The model under review builds one solid part; all positions refer to its coordinate system, in mm. Face numbers are marked on the shaded views. A direction names the side the tool comes from. Coordinates: 2 decimals unless noted, no trailing zeros. Order: outer loops, then holes, each group sorted by start corner. A loop starts at its lowest first (then second) coordinate and runs counter-clockwise, first axis right, second up.
```python
from build123d import *

# Parameters (mm, degrees)
F0_W     = 15
F0_H     = 9.5
F1_DEPTH = 22
F0_W_2   = 8.7
F0_H_2   = 2.8
F2_DEPTH = 12
F3_R     = 1.5


with BuildPart() as f1:
    # F0 (on Top) → F1 (new body)
    with BuildSketch(Plane.XY):
        with Locations((0, 0.571325)):
            Rectangle(F0_W, F0_H)
        Polygon((5.5, 2.5), (5.5, -2.5), (-5.5, -2.5), (-5.5, 2.5), (-1.25, 2.5), (-1.25, 4.012365), (1.25, 4.012365), (1.25, 2.5), align=None, mode=Mode.SUBTRACT)
    extrude(amount=F1_DEPTH)

    # F0 (on Top) → F2 (join)
    with BuildSketch(Plane.XY):
        Polygon((-5.5, -2.5), (5.5, -2.5), (5.5, 2.5), (1.25, 2.5), (1.25, 4.012365), (-1.25, 4.012365), (-1.25, 2.5), (-5.5, 2.5), align=None)
        Rectangle(F0_W_2, F0_H_2, mode=Mode.SUBTRACT)
    extrude(amount=F2_DEPTH)

    # F3
    f3_edges = [f1.edges().sort_by_distance(p)[0] for p in [
        (-7.5, 5.321325, 11),
        (7.5, 5.321325, 11),
        (7.5, -4.178675, 11),
        (-7.5, -4.178675, 11),
    ]]
    fillet(f3_edges, radius=F3_R)


solid = f1.part
```
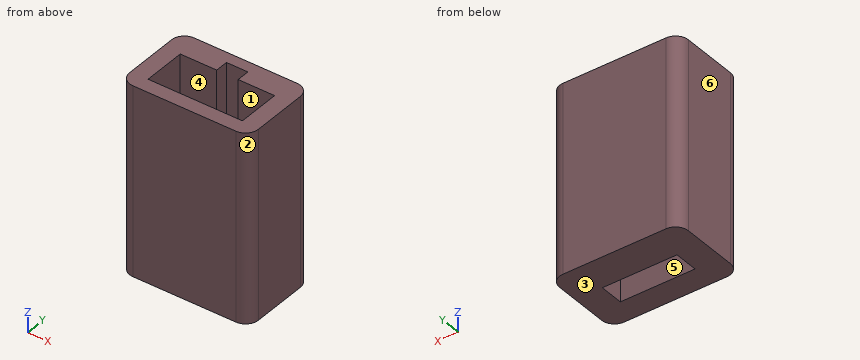
(1) We need section D-D, the plane y = 3. Write out the cut boundary in (x, z).
A:
outline: (-7.5, 0) - (7.5, 0) - (7.5, 22) - (1.25, 22) - (1.25, 12) - (-1.25, 12) - (-1.25, 22) - (-7.5, 22) - close
(2) Wall thickness on probe 1 along X at (y, z) = (-1.25, 14); probe 2 along Y at (x, z) = (-3.25, 11.5); probe 3 along Y at (x, z) = (-1.75, 20.75): over which ranges is each line inside the solid? List them lowest first.
A:
probe 1: x = -7.5 to -5.5, 5.5 to 7.5
probe 2: y = -4.18 to -1.4, 1.4 to 5.32
probe 3: y = -4.18 to -2.5, 2.5 to 5.32
(3) For pin 1 Ø3.5 at (x, y) = (1, 0) entering from +Z, flat-tipped, find the tip position at first contact; note if it passes through.
A:
pin 1: stops at z = 12
(4) Draft analysis for pull direction X (two halves, no side actions). For the marked faces 1, 2 and 3, state which applies: released by +X, released by -X, zero draft, split by the parting line, or undercut.
A:
face 1: undercut
face 2: released by +X
face 3: zero draft
(5) We need section A-A, the plane x = 1.5. Write out the cut boundary in (y, z), and give its area (3 significant figures).
A:
outline: (-4.18, 0) - (-1.4, 0) - (-1.4, 12) - (-2.5, 12) - (-2.5, 22) - (-4.18, 22) - close; (1.4, 0) - (5.32, 0) - (5.32, 22) - (2.5, 22) - (2.5, 12) - (1.4, 12) - close
area: 125 mm2
(6) Machinability: for the marked faces 4, 5 and 6, which of the approach directions +Z, -Z, +X, -X, +Y, -Y give a long, thin tool a straight path to every point of the face, cutting with its end or side? Answer none if there is none.
A:
face 4: +Z
face 5: +Z, -Z
face 6: +Z, -Z, -X, +Y, -Y
(7) We need section B-B, the plane z = 17.5. Write out the cut boundary in (x, y).
A:
outline: (-7.5, -2.68) arc R1.5 ccw to (-6, -4.18) - (6, -4.18) arc R1.5 ccw to (7.5, -2.68) - (7.5, 3.82) arc R1.5 ccw to (6, 5.32) - (-6, 5.32) arc R1.5 ccw to (-7.5, 3.82) - close; hole (-5.5, -2.5) - (5.5, -2.5) - (5.5, 2.5) - (1.25, 2.5) - (1.25, 4.01) - (-1.25, 4.01) - (-1.25, 2.5) - (-5.5, 2.5) - close
(8) We need section C-C, the plane y = -0.5. Write out the cut boundary in (x, z).
A:
outline: (-7.5, 0) - (-4.35, 0) - (-4.35, 12) - (-5.5, 12) - (-5.5, 22) - (-7.5, 22) - close; (4.35, 0) - (7.5, 0) - (7.5, 22) - (5.5, 22) - (5.5, 12) - (4.35, 12) - close
